Source: CAD feature listing. Evaluate the final solid. Frame: model axes, mm. A direction names the side the tool comes from. Give positions to 0.01 mm unless a question says otherwise; leave off trailing zeros. Order: outer loops, then holes, each group sorted by start corner. A loop starts at its lowest first (then second) coordinate and runs counter-clockwise, first axis right, second up. Notation, with made-up numbers: M -33.75,74 L 22.25,74 A8 ccw 22.25,83 Z; hole C -31.75,47 d7. An arc over 180 degrees is marked long. Answer as a JSON object with one key per item and string values. Group by question number.
1. Section query D-D (x = 38). Output: boundary loops of the cut face in (y, z), plus the area to 3 significant figures.
2. Material intervals for L1, parallel to Z at x = -12.5, y = 4.3; L2, parallel to Z at x = -6.5, y = 9.75; L3, parallel to Z at x = 27.5, y = 4.25, sorted ascending. Write a range as [from, to].
3. Pin query (flat end, axial travel): P1, Ø3, axis at y = 4.3, z = 48.37, coming from the +X side; P2, Ø2, axis at x = 10.5, z = 45, coming from the +Y side; P3, Ø3, axis at x = 36.5, z = 47, coming from the +Y side; P4, Ø2, axis at y = 4.3, z = 48.37, coming from the -X side. Return the tip coordinate at first contact, or that it passes through.
4. Section query B-B (y = 7). Output: boundary loops of the cut face in (x, z).
5. Section query A-A (x = -2). Output: boundary loops of the cut face in (y, z), plus the area to 3 significant figures.
6. Section query C-C (x = -28). Output: boundary loops of the cut face in (y, z), plus the area to 3 significant figures.
7. Set-up query: faces 4 (the flat face through (0, 6, -1)), 5 (the cylindrical face through (-45.1, 10.51, 42.14)), 6 (the flat face through (29.5, 6, 47)). Return all of +Z, -Z, +X, -X, +Y, -Y with unobstructed straight access to the full face (end or side cutting, diameter ignored); none if empty.
8. Pull-direction query (X, two-part tool) for faces 1 (the cylindrical face through (48.859, 1.203, -0.644)), 2 (the cylindrical face through (0.644, 1.203, 48.859)), 3 (the flat face through (40.5, 6, 47)); classes: +X half, -X half, draft (parallel to the pull), parting line (faces both ways), or undercut.
from build123d import *

# Parameters (mm, degrees)
SKETCH_1_W               = 100
SKETCH_1_H               = 100
EXTRUDE_1_DEPTH          = 9.5
FILLET_1_R               = 4
SKETCH_3_W               = 92
SKETCH_3_H               = 89
EXTRUDE_2_DEPTH          = 2
FILLET_2_R               = 3
SKETCH_2_W               = 11
SKETCH_2_H               = 7
CUT_EXTRUDE_1_DEPTH      = 8
SKETCH_4_R               = 1.25
CUT_EXTRUDE_2_DEPTH      = 91.5
CUT_EXTRUDE_2_DEPTH_BACK = 10.5
SKETCH_5_W               = 30
SKETCH_5_H               = 2
CUT_EXTRUDE_3_DEPTH      = 12.5


with BuildPart() as part:
    # Эскиз1 → Бобышка-Вытянуть1 (new body)
    with BuildSketch(Plane(origin=(0, 0, 0), x_dir=(1, 0, 0), z_dir=(0, 1, 0))):
        Rectangle(SKETCH_1_W, SKETCH_1_H)
    extrude(amount=EXTRUDE_1_DEPTH)

    # Скругление1
    fillet_1_edges = [part.edges().sort_by_distance(p)[0] for p in [
        (0, 0, 50),
        (-50, 0, 0),
        (0, 0, -50),
        (50, 0, 0),
        (50, 4.75, 50),
        (-50, 4.75, 50),
        (-50, 4.75, -50),
        (50, 4.75, -50),
    ]]
    fillet(fillet_1_edges, radius=FILLET_1_R)

    # Эскиз3 → Бобышка-Вытянуть2 (add)
    with BuildSketch(Plane(origin=(0, 9.5, 0), x_dir=(1, 0, 0), z_dir=(0, 1, 0))):
        with Locations((0, 1.5)):
            Rectangle(SKETCH_3_W, SKETCH_3_H)
    extrude(amount=EXTRUDE_2_DEPTH)

    # Скругление2
    fillet_2_edges = [part.edges().sort_by_distance(p)[0] for p in [
        (46, 10.5, 43),
        (46, 10.5, -46),
        (-46, 10.5, -46),
        (-46, 10.5, 43),
    ]]
    fillet(fillet_2_edges, radius=FILLET_2_R)

    # Эскиз2 → Вырез-Вытянуть1 (cut)
    with BuildSketch(Plane(origin=(0, 9.5, 0), x_dir=(1, 0, 0), z_dir=(0, 1, 0))):
        with Locations((35, -46.5)):
            Rectangle(SKETCH_2_W, SKETCH_2_H)
        with Locations((-35, -46.5)):
            Rectangle(SKETCH_2_W, SKETCH_2_H)
    extrude(amount=-CUT_EXTRUDE_1_DEPTH, mode=Mode.SUBTRACT)

    # Эскиз4 → Вырез-Вытянуть2 (cut, two sides)
    with BuildSketch(Plane(origin=(-40.5, 0, 0), x_dir=(0, 0, -1), z_dir=(1, 0, 0))) as cut_extrude_2_sk:
        with Locations((-48.37, 4.3)):
            Circle(SKETCH_4_R)
    extrude(amount=CUT_EXTRUDE_2_DEPTH, mode=Mode.SUBTRACT)
    extrude(cut_extrude_2_sk.sketch, amount=-CUT_EXTRUDE_2_DEPTH_BACK, mode=Mode.SUBTRACT)

    # Эскиз5 → Вырез-Вытянуть3 (cut, through all)
    with BuildSketch(Plane.XZ):
        Rectangle(SKETCH_5_W, SKETCH_5_H)
    extrude(amount=-CUT_EXTRUDE_3_DEPTH, mode=Mode.SUBTRACT)


solid = part.part
Answer sheet:
{
 "1": {"outline": "M 0,-46 A4 ccw 4,-50 L 9.5,-50 L 9.5,-46 L 11.5,-46 L 11.5,43 L 1.5,43 L 1.5,49.12 A4 ccw 0,46 Z", "area": "1,070 mm^2"},
 "2": {"L1": "[-50, -1], [1, 47.12], [49.62, 50]", "L2": "[-46, -1], [1, 43]", "L3": "[-50, 47.12], [49.62, 50]"},
 "3": {"P1": "x = 49.9", "P2": "y = 9.5", "P3": "y = 1.5", "P4": "through"},
 "4": {"outline": "M -50,-46 A4 ccw -46,-50 L 46,-50 A4 ccw 50,-46 L 50,46 A4 ccw 46,50 L 40.5,50 L 40.5,43 L 29.5,43 L 29.5,50 L -29.5,50 L -29.5,43 L -40.5,43 L -40.5,50 L -46,50 A4 ccw -50,46 Z; hole M -15,-1 L 15,-1 L 15,1 L -15,1 Z"},
 "5": {"outline": "M 0,-46 A4 ccw 4,-50 L 9.5,-50 L 9.5,-46 L 11.5,-46 L 11.5,-1 L 0,-1 Z; M 0,1 L 11.5,1 L 11.5,43 L 9.5,43 L 9.5,50 L 4,50 A4 ccw 0,46 Z; hole C 4.3,48.37 d2.5", "area": "1,090 mm^2"},
 "6": {"outline": "M 0,-46 A4 ccw 4,-50 L 9.5,-50 L 9.5,-46 L 11.5,-46 L 11.5,43 L 9.5,43 L 9.5,50 L 4,50 A4 ccw 0,46 Z; hole C 4.3,48.37 d2.5", "area": "1,120 mm^2"},
 "7": {"face 4": "+Y, -Y", "face 5": "+Z, -X, +Y", "face 6": "+Z, +Y"},
 "8": {"face 1": "+X half", "face 2": "draft", "face 3": "undercut"}
}
